Source: three-view drawing plus pictorial views. Frame: mm from the lowest corner of the part. Round coordinates to 2 decimals unless told otherwise and drop trailing zeros. Write each loop counter-clockwise with the first axis right and the second up, starting at its lowest first coordinate (ties: lowest second). Pieces come first, ordered by that corner, then holes. Notation, with made-up numbers: (-33, -1.5) -> (-8, -1.5) arc R14 ccw to (-8, 11.5) -> close; hole circle Ø11 at (51, -24). An arc over 180 degrees is marked (long way). Put each result on its own line as item: value.
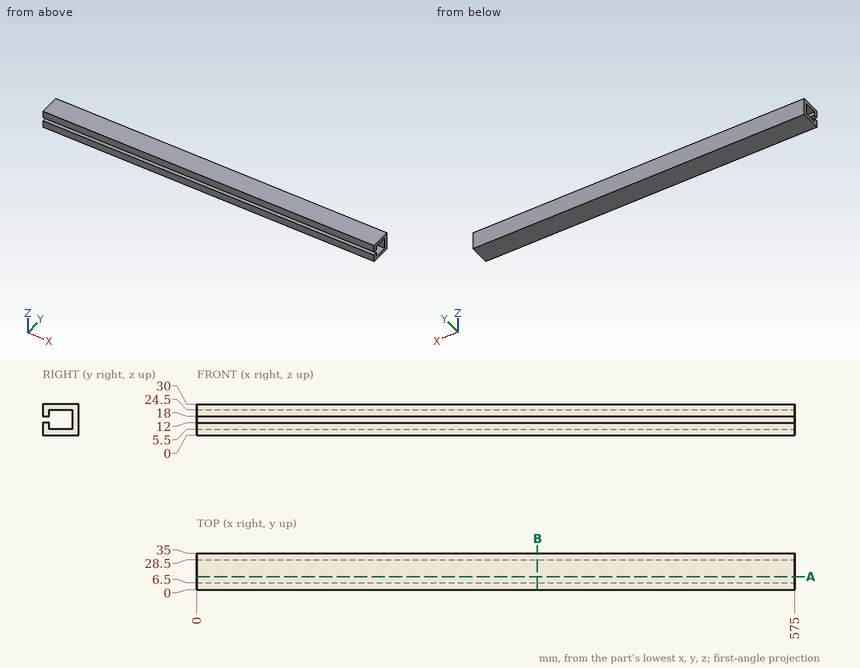
Q1. Pin query (flat end, axial travel): pin 1 (1 mm diameter, centred on x = 306, z = 13.5, fed in from -Y). Return the tip coordinate at first contact, or that it passes through.
Ans:
pin 1: stops at y = 28.5
Q2. Material intervals for line 1 (Z direction, x = 264.5, y = 13); line 2 (Z direction, x = 447.5, y = 2); line 3 (Y direction, x = 108, z = 10), sorted ascending. Write a range as [from, to].
Ans:
line 1: z = [0, 5.5], [24.5, 30]
line 2: z = [0, 12], [18, 30]
line 3: y = [0, 6.5], [28.5, 35]
Q3. Cut plane B-B on x = 327.5. Output: boundary loops of the cut face in (y, z).
Ans:
outline: (0, 0) -> (35, 0) -> (35, 30) -> (0, 30) -> (0, 18) -> (6.5, 18) -> (6.5, 24.5) -> (28.5, 24.5) -> (28.5, 5.5) -> (6.5, 5.5) -> (6.5, 12) -> (0, 12) -> close
Q4. Cut plane A-A on y = 12.5. Output: boundary loops of the cut face in (x, z).
Ans:
outline: (0, 0) -> (575, 0) -> (575, 5.5) -> (0, 5.5) -> close; (0, 24.5) -> (575, 24.5) -> (575, 30) -> (0, 30) -> close
